Check sheet for the modelled part. Datum: model origin and axes. Units: mm. A direction names the side the tool comes from. Round coordinates to 2 decimals unless told otherwise and drop trailing zeros. Write each loop counter-clockwise with the first axis right and the second up, starting at its lowest first coordinate (ties: lowest second). Pieces come first, ordered by that corner, then holes. Notation, with made-up numbers: M 30,-32 L 62,-32 A25 cw 62,-5 Z; hole C -22,5.5 d3. An arc over 180 degrees is marked long. Answer in a Markdown table with one row per item.
```python
from build123d import *

# Parameters (mm, degrees)
F2_ANGLE       = 30
F3_DEPTH       = 25.4
F4_R           = 0.635
F6_D           = 6.35
F6_CSINK_D     = 12.7
F6_CSINK_ANGLE = 90


with BuildPart() as f2:
    # F0 (on Top) → F2 (revolve)
    with BuildSketch(Plane.XY):
        Polygon((21.0717357695, -15.9602742642), (21.0717357695, 15.9602742642), (-21.0717357695, 15.9602742642), (-21.0717357695, -15.9602742642), (-0.2086274326, -15.9602742642), (-0.2086274326, -17.420691438), (16.899112612, -17.420691438), (16.899112612, -15.9602742642), align=None)
    revolve(axis=Axis((-61.1288920045, 1.6690483317, 0), (0, -1, 0)), revolution_arc=F2_ANGLE)

    # F3 (add): a face of the model
    f3_faces = [f2.faces().sort_by_distance(p)[0] for p in [
        (-8.057939505, -0.3043307955, 30.6405287117),
    ]]
    extrude(f3_faces, amount=F3_DEPTH)

    # F4
    f4_edges = [f2.edges().sort_by_distance(p)[0] for p in [
        (-2.284435, -15.960274, 15.767325),
        (-14.720395, -15.960274, 41.458655),
    ]]
    fillet(f4_edges, radius=F4_R)

    # F6 (through all)
    with Locations(Plane.XZ.offset(17.420691438)):
        with Locations((7.227263879, 10.6254266575), (3.5499625374, 24.5596691966), (-3.6885414738, 40.8757403493)):
            CounterSinkHole(F6_D / 2, F6_CSINK_D / 2, counter_sink_angle=F6_CSINK_ANGLE)


solid = f2.part
```
1. Section check B-B, the plane z = 55.5. Record the cut outline in (x, y), and give its area (3 significant figures).
Found:
| item | result |
|---|---|
| outline | M -15.8,-17.42 L -3.07,-17.42 L -3.07,-15.96 L 1.75,-15.96 L 1.75,15.96 L -15.8,15.96 Z |
| area | 579 mm2 |
2. Access from +Z, -Z, +X, -X, +Y, -Y to the whole of each face (thin tool, end or side, straight path). Record for faces 5 (the face through (-2.227, -17.014, 15.552)), 6 (the face through (0.184, -16.701, 49.859)), 7 (the face through (2.085, 1.069, 21.743)).
Found:
| item | result |
|---|---|
| face 5 | -Z, -X, -Y |
| face 6 | +Z, +X, -Y |
| face 7 | +Y, -Y |
3. Draft check along Z on faces 1 (the face through (0, 0, 0)), 2 (the face through (-10, 15.96, 29)), 3 (the face through (3.98, -14.4, 27.86)), 4 (the face through (4.052, -14.4, 11.625)). Enter one of: +Z half, -Z half, draft (parallel to the pull), parting line (faces both ways), or undercut.
Found:
| item | result |
|---|---|
| face 1 | -Z half |
| face 2 | draft |
| face 3 | undercut |
| face 4 | undercut |
4. Scan lines: L1, parallel to Y at x = -27.5, z = 47; L2, parallel to X at y = 11.5, z = 10.5; L3, parallel to X at y = -1.5, z = 8. Record each from-to range of solid material in increasing order.
Found:
| item | result |
|---|---|
| L1 | y = -15.96 to 15.96 |
| L2 | x = -22.47 to 4.05, 10.4 to 20.4 |
| L3 | x = -21.88 to 5.44, 9.01 to 20.68 |
5. Go/stop test with flat-tipped pins: pin 1 (2 mm diameter, centred on y = 4, z = 15, fed in from +X); pin 2 (19 mm diameter, centred on x = -29, z = 14, fed in from -Y); pin 3 (12 mm diameter, centred on y = 2, z = 34, fed in from -X). Record where each tip stops, or that it passes through.
Found:
| item | result |
|---|---|
| pin 1 | stops at x = 19.87 |
| pin 2 | stops at y = -15.96 |
| pin 3 | stops at x = -37.97 |
6. Section check C-C, the plane x = -33. Record the cut outline in (y, z).
Found:
| item | result |
|---|---|
| outline | M -15.96,31.39 L 15.96,31.39 L 15.96,45.57 L -15.96,45.57 Z |
7. Section check A-A, the plane y = -4. Record the cut outline in (x, z) (3 decimals), and give its area (3 significant figures).
Found:
| item | result |
|---|---|
| outline | M -39.138,42.026 L -26.438,20.029 A40.057 cw -21.072,0 L 21.072,0 A82.201 ccw 10.059,41.1 L -2.641,63.097 Z; hole C -3.689,40.876 d6.35; hole C 3.55,24.56 d6.35; hole C 7.227,10.625 d6.35 |
| area | 2,320 mm2 |
